Check sheet for the modelled part. Datum: model origin and axes. Units: mm. A direction names the side the tool comes from. Give positions to 0.01 mm unless a question says otherwise; leave off trailing zeros. Loops run counter-clockwise (first coordinate to the right, second up) from the corner with the lowest first, then second, coordinate; pieces in that order, holes last. Notation, with made-up numbers: (2.5, 70.5) - (34.5, 70.5) arc R16 ccw to (34.5, 87.5) - close; hole circle Ø1 at (33.5, 67). An arc over 180 degrees is marked (long way). Use CSV: the item, a comma, the result in double quotes.
from build123d import *

# Parameters (mm, degrees)
SKETCH1_R           = 2
BOSS_EXTRUDE1_DEPTH = 5
FILLET1_R           = 2


with BuildPart() as part:
    # Sketch1 → Boss-Extrude1 (new body)
    with BuildSketch(Plane.XY):
        with BuildLine():
            Line((8, 4), (-8, 4))
            Line((-8, 4), (-8, -4))
            Line((-8, -4), (8, -4))
            Line((8, -4), (8, -2.5))
            Line((8, -2.5), (14.377501001, -2.5))
            ThreePointArc((14.377501001, -2.5), (21.5, 0), (14.377501001, 2.5))
            Line((14.377501001, 2.5), (8, 2.5))
            Line((8, 2.5), (8, 4))
        make_face()
        with Locations((-4, 0)):
            Circle(SKETCH1_R, mode=Mode.SUBTRACT)
        with Locations((4, 0)):
            Circle(SKETCH1_R, mode=Mode.SUBTRACT)
        with BuildLine():
            ThreePointArc((20, 0), (17.5, -2.5), (15, 0))
            ThreePointArc((15, 0), (17.5, 2.5), (20, 0))
        make_face(mode=Mode.SUBTRACT)
    extrude(amount=BOSS_EXTRUDE1_DEPTH)

    # Fillet1
    # the kernel refuses this fillet: 2 mm, written as the material it adds along each edge
    with BuildSketch(Plane(origin=(14.377501001, -2.5, 0), x_dir=(0.6900779887780536, -0.7237350132500407, 0), z_dir=(0, 0, 1))) as fillet1_piece_1:
        with BuildLine():
            CenterArc((0.863575741, -1.992528413), FILLET1_R, 94.954095219, 41.409622109)
            Line((-0.583894286, -0.612372436), (-0.612843687, -0.584769316))
            Line((-0.612843687, -0.584769316), (-0.028949401, 0.02760312))
            Line((-0.028949401, 0.02760312), (0.003454303, 0.039850568))
            ThreePointArc((0.003454303, 0.039850568), (0.345430296, 0.025056827), (0.687406289, 0.039850568))
            Line((0.687406289, 0.039850568), (0.690860592, 0))
        make_face()
    extrude(amount=5)
    with BuildSketch(Plane(origin=(8, -2.5, 0), x_dir=(1, 0, 0), z_dir=(0, 0, 1))) as fillet1_piece_2:
        with BuildLine():
            CenterArc((1.936491673, -2), FILLET1_R, 90, 75.522487814)
            Line((0, -1.5), (-0.038729833, -1.49))
            ThreePointArc((-0.038729833, -1.49), (-0.04, -0.75), (-0.04, 0))
            Line((-0.04, 0), (0, 0.04))
            Line((0, 0.04), (1.936491673, 0.04))
            Line((1.936491673, 0.04), (1.936491673, 0))
        make_face()
    extrude(amount=5)
    with BuildSketch(Plane(origin=(14.377501001, 2.5, 0), x_dir=(0.6900779887780526, 0.7237350132500416, 0), z_dir=(0, 0, 1))) as fillet1_piece_3:
        with BuildLine():
            CenterArc((0.863575741, 1.992528413), FILLET1_R, 223.636282672, 41.409622109)
            Line((-0.583894286, 0.612372436), (-0.612843687, 0.584769316))
            Line((-0.612843687, 0.584769316), (-0.028949401, -0.02760312))
            Line((-0.028949401, -0.02760312), (0.003454303, -0.039850568))
            ThreePointArc((0.003454303, -0.039850568), (0.345430296, -0.025056827), (0.687406289, -0.039850568))
            Line((0.687406289, -0.039850568), (0.690860592, 0))
        make_face()
    extrude(amount=5)
    with BuildSketch(Plane(origin=(8, 2.5, 0), x_dir=(0, 1, 0), z_dir=(0, 0, 1))) as fillet1_piece_4:
        with BuildLine():
            CenterArc((2, -1.936491673), FILLET1_R, 104.477512186, 75.522487814)
            Line((0, -1.936491673), (-0.04, -1.936491673))
            Line((-0.04, -1.936491673), (-0.04, 0))
            Line((-0.04, 0), (0, 0.04))
            ThreePointArc((0, 0.04), (0.75, 0.04), (1.49, 0.038729833))
            Line((1.49, 0.038729833), (1.5, 0))
        make_face()
    extrude(amount=5)


solid = part.part
1. Sectioned sample at C-C, the plane z = 3.4. Record the boundary of the cut face in (x, y), and give its area (3 significant figures).
Completed:
outline,"(-8, -4) - (8, -4) arc R2 cw to (9.94, -2.5) - (13.53, -2.5) arc R2 cw to (14.85, -3) arc R4 ccw (long way) to (14.85, 3) arc R2 cw to (13.53, 2.5) - (9.94, 2.5) arc R2 cw to (8, 4) - (-8, 4) - close; hole circle Ø4 at (-4, 0); hole circle Ø4 at (4, 0); hole circle Ø5 at (17.5, 0)"
area,"164 mm²"
2. Go/stop test with flat-tipped pins: pin 1 Ø1.5 at (x, z) = (12, 1.5) entering from -Y; pin 2 Ø3 at (y, z) = (2, 3) entering from +X; pin 3 Ø2.5 at (x, y) = (-4, 0) entering from -Z; pin 4 Ø3 at (x, y) = (5, 1) entering from +Z. Record where each tip stops, or that it passes through.
Completed:
pin 1,"stops at y = -2.5"
pin 2,"stops at x = 21.47"
pin 3,"passes through"
pin 4,"stops at z = 5"
3. Sectioned sample at D-D, the plane y = 2.25. Record the boundary of the cut face in (x, z), and give its area (3 significant figures).
Completed:
outline,"(-8, 0) - (16.41, 0) - (16.41, 5) - (-8, 5) - close; (18.59, 0) - (20.81, 0) - (20.81, 5) - (18.59, 5) - close"
area,"133 mm²"
4. Sectioned sample at A-A, the plane x = 17.5. Record the boundary of the cut face in (y, z), and give its area (3 significant figures).
Completed:
outline,"(-4, 0) - (-2.5, 0) - (-2.5, 5) - (-4, 5) - close; (2.5, 0) - (4, 0) - (4, 5) - (2.5, 5) - close"
area,"15.0 mm²"
5. Sectioned sample at B-B, the plane y = 0. Record the boundary of the cut face in (x, z), and give its area (3 significant figures).
Completed:
outline,"(-8, 0) - (-6, 0) - (-6, 5) - (-8, 5) - close; (-2, 0) - (2, 0) - (2, 5) - (-2, 5) - close; (6, 0) - (15, 0) - (15, 5) - (6, 5) - close; (20, 0) - (21.5, 0) - (21.5, 5) - (20, 5) - close"
area,"82.5 mm²"
6. Scan lines: line 1 along Y through (x, z) = (-4, 2.8); line 2 along Y through (x, z) = (17.5, 3.7); line 3 along X through (y, z) = (-1.5, 2.75). Record each from-to range of solid material in increasing order.
Completed:
line 1,"y = -4 to -2, 2 to 4"
line 2,"y = -4 to -2.5, 2.5 to 4"
line 3,"x = -8 to -5.32, -2.68 to 2.68, 5.32 to 15.5, 19.5 to 21.21"
7. Set-up check for faces 4 (the face through (14.248, -2.633, 2.465)), 5 (the face through (21.5, -0.1, 2.5)), 6 (the face through (12, 2.5, 2)): record each of +Z, -Z, +X, -X, +Y, -Y from which the full face is reachable in a straight line by a thin tool's end or side.
Completed:
face 4,"+Z, -Z, -Y"
face 5,"+Z, -Z"
face 6,"+Z, -Z, +Y"
8. Release check for a two-part mould opening along X. For faces 1 (the face through (-5.6, -1.2, 2.5)), 2 (the face through (-8, 0, 2)), 3 (the face through (0, 4, 2)) record: released by +X, released by -X, zero draft, split by the parting line, or undercut.
Completed:
face 1,"undercut"
face 2,"released by -X"
face 3,"zero draft"
